```python
from build123d import *

# Parameters (mm, degrees)
SKETCH_1_W      = 45.5
SKETCH_1_H      = 97.5
EXTRUDE_1_DEPTH = 52.5
SKETCH_3_W      = 5
SKETCH_3_H      = 1


with BuildPart() as part:
    # 草图1 → 拉伸1 (new body)
    with BuildSketch(Plane(origin=(0, 0, 0), x_dir=(1, 0, 0), z_dir=(0, 1, 0))):
        Rectangle(SKETCH_1_W, SKETCH_1_H)
    extrude(amount=EXTRUDE_1_DEPTH)

    # 扫描1: sweep along a path in 草图4
    with BuildLine(Plane.ZY.offset(18.75)) as sweep_1_path:
        Line((-38.75, 52.5), (-38.75, 57.5))
        Line((-38.75, 57.5), (-28.75, 57.5))
    # 草图3 → 扫描1 (sweep)
    with BuildSketch(Plane(origin=(0, 52.5, 0), x_dir=(-1, 0, 0), z_dir=(0, 1, 0))):
        with Locations((16.25, -38.25)):
            Rectangle(SKETCH_3_W, SKETCH_3_H)
    sweep_1 = sweep(path=sweep_1_path.line, transition=Transition.RIGHT)

    # 镜向2: 扫描1 across plane
    add(sweep_1.mirror(Plane.ZY))


solid = part.part
```
Could you check a few things on this model? Use its own coordinates, in mm. A direction names the side the tool comes from. Round coordinates to 2 decimals unless told otherwise and drop trailing zeros. Loops run counter-clockwise (first coordinate to the right, second up) from the corner with the lowest first, then second, coordinate; pieces in that order, holes last.
Q1. I want a section at A-A (z = -32.5). Write out the boundary of the cut face in (x, y).
Q2. Thinking about a two-plate mould opening in Y: for faces 1 (the flat face through (16, 55, -38.75)), 2 (the flat face through (-16, 55, -37.75)), 3 (the flat face through (-16, 57.5, -34)), which applies, pulls with the +Y half, pulls with the -Y half, needs draft (parallel to the pull), parting line crosses it, or undercut?
Q3. Please list where these lines run through material, in increasing order: L1, parallel to Y at x = -11, z = -29; L2, parallel to Y at x = 14, z = -31.5.
Q4. I want a section at D-D (x = 3.5). Write out the boundary of the cut face in (y, z).
Q5. For P1, Ø1.5, axis at x = 15.5, y = 55.5, coming from the -Z side; P2, Ø0.5, axis at x = 17, y = 57, coming from the +Z side; P3, Ø8, axis at x = -14.5, z = -6.5, coming from the +Y side, each with a flat end and sliding along its axis, tell me the tip position at first contact or that it passes through.
Q6. I want a section at C-C (z = -9.5). Write out the boundary of the cut face in (x, y), and give its area (3 significant figures).
Q7. I want a section at B-B (x = -15). Write out the boundary of the cut face in (y, z).
Q8. On a 3-axis mill with a long thin cutter (end or side, diameter ignored), from which of +Z, -Z, +X, -X, +Y, -Y can I reach the whole of each face in a straight line? I mean faces 4 (the flat face through (16, 55, -37.75)), 5 (the flat face through (18.75, 57, -35)), 6 (the flat face through (-16, 55, -38.75)), 7 (the flat face through (-13.75, 57, -35)). Say none if no direction works.
Answer below:
1. outline: (-22.75, 0) - (22.75, 0) - (22.75, 52.5) - (-22.75, 52.5) - close; (-18.75, 56.5) - (-13.75, 56.5) - (-13.75, 57.5) - (-18.75, 57.5) - close; (13.75, 56.5) - (18.75, 56.5) - (18.75, 57.5) - (13.75, 57.5) - close
2. face 1: needs draft
2. face 2: undercut
2. face 3: pulls with the +Y half
3. L1: y = 0 to 52.5
3. L2: y = 0 to 52.5, 56.5 to 57.5
4. outline: (0, -48.75) - (52.5, -48.75) - (52.5, 48.75) - (0, 48.75) - close
5. P1: stops at z = -38.75
5. P2: stops at z = -28.75
5. P3: stops at y = 52.5
6. outline: (-22.75, 0) - (22.75, 0) - (22.75, 52.5) - (-22.75, 52.5) - close
6. area: 2,390 mm2
7. outline: (0, -48.75) - (52.5, -48.75) - (52.5, -38.75) - (57.5, -38.75) - (57.5, -28.75) - (56.5, -28.75) - (56.5, -37.75) - (52.5, -37.75) - (52.5, 48.75) - (0, 48.75) - close
8. face 4: +Z, +X, -X
8. face 5: +Z, -Z, +X, +Y
8. face 6: -Z, +X, -X, +Y
8. face 7: +Z, -Z, +Y
